```python
from build123d import *

# Parameters (mm, degrees)
SKETCH1_W                   = 158.75
SKETCH1_H                   = 38.1
BOSS_EXTRUDE1_DEPTH         = 1.6002
F_27_0_144_DIAMETER_HOLE1_D = 3.6576
F_1_2_0_5_DIAMETER_HOLE1_D  = 12.7
F_0_257_DIAMETER_HOLE1_D    = 6.5278
CHAMFER1_SIZE               = 2.54
CHAMFER2_SIZE               = 12.7


with BuildPart() as part:
    # Sketch1 → Boss-Extrude1 (new body)
    with BuildSketch(Plane(origin=(0, 0, 0), x_dir=(1, 0, 0), z_dir=(0, 1, 0))):
        with Locations((79.375, 19.05)):
            Rectangle(SKETCH1_W, SKETCH1_H)
    extrude(amount=BOSS_EXTRUDE1_DEPTH)

    # #27 (0.144) Diameter Hole1 (through all)
    with Locations(Plane(origin=(0, 1.6002, 0), x_dir=(1, 0, 0), z_dir=(0, 1, 0))):
        with Locations((5.785202787, 19.614797213), (19.614797213, 5.785202787), (5.785202787, 5.785202787), (19.614797213, 19.614797213), (152.964797213, 5.785202787), (139.135202787, 5.785202787), (139.135202787, 19.614797213), (152.964797213, 19.614797213)):
            Hole(F_27_0_144_DIAMETER_HOLE1_D / 2)

    # 1/2 (0.5) Diameter Hole1 (through all)
    with Locations(Plane(origin=(0, 1.6002, 0), x_dir=(1, 0, 0), z_dir=(0, 1, 0))):
        with Locations((12.7, 12.7), (146.05, 12.7)):
            Hole(F_1_2_0_5_DIAMETER_HOLE1_D / 2)

    # F (0.257) Diameter Hole1 (through all)
    with Locations(Plane(origin=(0, 1.6002, 0), x_dir=(1, 0, 0), z_dir=(0, 1, 0))):
        with Locations((53.975, 31.75), (104.775, 31.75)):
            Hole(F_0_257_DIAMETER_HOLE1_D / 2)

    # Chamfer1
    chamfer1_edges = [part.edges().sort_by_distance(p)[0] for p in [
        (158.75, 0.8001, 0),
        (0, 0.8001, 0),
    ]]
    chamfer(chamfer1_edges, length=CHAMFER1_SIZE)

    # Chamfer2
    chamfer2_edges = [part.edges().sort_by_distance(p)[0] for p in [
        (0, 0.8001, -38.1),
        (158.75, 0.8001, -38.1),
    ]]
    chamfer(chamfer2_edges, length=CHAMFER2_SIZE)


solid = part.part
```
Check sheet for the modelled part. Datum: model origin and axes. Units: mm. Coordinates: 2 decimals unless noted, no trailing zeros. Loops run counter-clockwise (first coordinate to the right, second up) from the corner with the lowest first, then second, coordinate; pieces in that order, holes last. Notation, with made-up numbers: M -27.75,-4.5 L 14.25,-4.5 A25 cw 14.25,7.5 Z; hole C 58.5,63.25 d1. An arc over 180 degrees is marked long. Answer as a JSON object with one key per item and string values.
1. Sectioned sample at B-B on y = 1.05. Count the separate pieces of the cut face and the enclosed holes in it, and give its area (3 significant figures).
Outcome:
{"separate pieces": "1", "enclosed holes": "12", "area": "5,480 mm²"}
2. Scan lines: L1, parallel to X at y = 0.65, z = -5.5; L2, parallel to X at y = 1, z = -5; L3, parallel to Z at x = 146.05, y = 0.95. Record each from-to range of solid material in increasing order. Write a range as from..to.
Outcome:
{"L1": "0..3.98, 7.59..17.81, 21.42..137.33, 140.94..151.16, 154.77..158.75", "L2": "0..4.13, 7.44..17.96, 21.27..137.48, 140.79..151.31, 154.62..158.75", "L3": "-38.1..-19.05, -6.35..0"}
3. Sectioned sample at A-A on z = -12.7. Record the cut outline in (x, y), and give its area (3 significant figures).
Outcome:
{"outline": "M 0,0 L 6.35,0 L 6.35,1.6 L 0,1.6 Z; M 19.05,0 L 139.7,0 L 139.7,1.6 L 19.05,1.6 Z; M 152.4,0 L 158.75,0 L 158.75,1.6 L 152.4,1.6 Z", "area": "213 mm²"}
4. Release check for a two-part mould opening along X. For faces 1 (the cylindrical face through (6.02, 0.79, -21.43)), 2 (the flat face through (78, 1.6, -19)), 3 (the flat face through (157.5, 0.79, -1.29)) record: pulls with the +X half, pulls with the -X half, needs draft (parallel to the pull), parting line crosses it, or undercut.
Outcome:
{"face 1": "undercut", "face 2": "needs draft", "face 3": "pulls with the +X half"}
5. Sectioned sample at C-C on z = -31.75. Record the cut outline in (x, y), and give its area (3 significant figures).
Outcome:
{"outline": "M 6.35,0 L 50.71,0 L 50.71,1.6 L 6.35,1.6 Z; M 57.24,0 L 101.51,0 L 101.51,1.6 L 57.24,1.6 Z; M 108.04,0 L 152.4,0 L 152.4,1.6 L 108.04,1.6 Z", "area": "213 mm²"}
6. Depth check by flat-ended pin: P1, Ø2, axis at x = 139.14, z = -5.79, coming from the +Y side. Enter the tip coordinate at first touch or a pass-through.
Outcome:
{"P1": "through"}
